```python
from build123d import *

# Parameters (mm, degrees)
SKETCH1_R               = 22
BOSS_EXTRUDE1_DEPTH     = 8.25
SKETCH2_R               = 18
CUT_EXTRUDE1_DEPTH      = 13.5
SKETCH3_R               = 19.5
CUT_EXTRUDE2_DEPTH      = 8
CUT_EXTRUDE3_DEPTH      = 36.217183306
CUT_EXTRUDE3_DEPTH_BACK = 36.217183306
SKETCH4_R               = 10
SKETCH6_W               = 3.4
SKETCH6_H               = 2.2
CUT_EXTRUDE5_DEPTH      = 8
CIRPATTERN1_COUNT       = 4
CUT_EXTRUDE6_START      = -1.5
SKETCH7_R               = 22
CUT_EXTRUDE6_DEPTH      = 1.5
CHAMFER1_SIZE           = 1
BOSS_EXTRUDE2_START     = 5
BOSS_EXTRUDE2_DEPTH     = 5
SKETCH9_W               = 10
SKETCH9_H               = 5
CUT_EXTRUDE7_DEPTH      = 37.986484018
SKETCH10_R              = 1
CUT_EXTRUDE8_DEPTH      = 42.764967377


with BuildPart() as part:
    # Sketch1 → Boss-Extrude1 (new, symmetric)
    with BuildSketch(Plane.XY):
        Circle(SKETCH1_R)
    extrude(amount=BOSS_EXTRUDE1_DEPTH, both=True)

    # Sketch2 → Cut-Extrude1 (cut)
    with BuildSketch(Plane.XY.offset(8.25)):
        Circle(SKETCH2_R)
    extrude(amount=-CUT_EXTRUDE1_DEPTH, mode=Mode.SUBTRACT)

    # Sketch3 → Cut-Extrude2 (cut)
    with BuildSketch(Plane.XY.offset(8.25)):
        Circle(SKETCH3_R)
    extrude(amount=-CUT_EXTRUDE2_DEPTH, mode=Mode.SUBTRACT)

    # Sketch4 → Cut-Extrude3 (cut, two sides: drawn at the far end of the back side and taken through both)
    with BuildSketch(Plane(origin=(0, 0, -8.25), x_dir=(-1, 0, 0), z_dir=(0, 0, -1)).offset(-CUT_EXTRUDE3_DEPTH_BACK)):
        with Locations(Location((0, 0, 0), (0, 0, 180))):
            Circle(SKETCH4_R)
    extrude(amount=CUT_EXTRUDE3_DEPTH + CUT_EXTRUDE3_DEPTH_BACK, mode=Mode.SUBTRACT)

    # Sketch6 → Cut-Extrude5 (cut)
    with BuildSketch(Plane.XY.offset(8.25)):
        with Locations((0, 19.5)):
            Rectangle(SKETCH6_W, SKETCH6_H)
    cut_extrude5 = extrude(amount=-CUT_EXTRUDE5_DEPTH, mode=Mode.SUBTRACT)

    # CirPattern1: Cut-Extrude5 ×4 about axis
    cirpattern1_axis = Axis((0, 0, 0), (0, 0, 1))
    for i in range(1, CIRPATTERN1_COUNT):
        add(cut_extrude5.rotate(cirpattern1_axis, i * 360 / CIRPATTERN1_COUNT), mode=Mode.SUBTRACT)

    # Sketch7 → Cut-Extrude6 (cut)
    with BuildSketch(Plane(origin=(0, 0, -8.25), x_dir=(-1, 0, 0), z_dir=(0, 0, -1)).offset(CUT_EXTRUDE6_START)):
        Circle(SKETCH7_R)
    extrude(amount=CUT_EXTRUDE6_DEPTH, mode=Mode.SUBTRACT)

    # Chamfer1
    chamfer1_edges = [part.edges().sort_by_distance(p)[0] for p in [
        (-22, 0, 8.25),
    ]]
    chamfer(chamfer1_edges, length=CHAMFER1_SIZE)

    # Sketch8 → Boss-Extrude2 (add)
    with BuildSketch(Plane(origin=(0, 0, -6.75), x_dir=(-1, 0, 0), z_dir=(0, 0, -1)).offset(BOSS_EXTRUDE2_START)):
        with BuildLine():
            Line((5, 9), (5, 11.5))
            Line((5, 11.5), (10, 11.5))
            Line((10, 11.5), (10, 15.5))
            Line((10, 15.5), (-10, 15.5))
            Line((-10, 15.5), (-10, 11.5))
            Line((-10, 11.5), (-5, 11.5))
            Line((-5, 11.5), (-5, 9))
            Line((-5, 9), (-4.358898944, 9))
            ThreePointArc((-4.358898944, 9), (0, 10), (4.358898944, 9))
            Line((4.358898944, 9), (5, 9))
        make_face()
    extrude(amount=-BOSS_EXTRUDE2_DEPTH)

    # Sketch9 → Cut-Extrude7 (cut, through all)
    with BuildSketch(Plane(origin=(0, 0, -11.75), x_dir=(-1, 0, 0), z_dir=(0, 0, -1))):
        with Locations((0, 11)):
            Rectangle(SKETCH9_W, SKETCH9_H)
    extrude(amount=-CUT_EXTRUDE7_DEPTH, mode=Mode.SUBTRACT)

    # Sketch10 → Cut-Extrude8 (cut, through all)
    with BuildSketch(Plane.XZ.offset(-11.5)):
        with Locations(Location((-7.5, -9.25, 0), (0, 0, 270))):
            Circle(SKETCH10_R)
        with Locations(Location((7.5, -9.25, 0), (0, 0, 180))):
            Circle(SKETCH10_R)
    extrude(amount=-CUT_EXTRUDE8_DEPTH, mode=Mode.SUBTRACT)


solid = part.part
```
CAD build for the part. Positions are in the model's coordinates, mm. A direction names the side the tool comes from. Round coordinates to 2 decimals unless told otherwise and drop trailing zeros. Loops run counter-clockwise (first coordinate to the right, second up) from the corner with the lowest first, then second, coordinate; pieces in that order, holes last. Notation, with made-up numbers: M 14.25,1 L 32.25,1 A13 cw 32.25,12 Z; hole C -37.75,-26.5 d7. An arc over 180 degrees is marked long. Return JSON: item names as keys, results as strings. Group by question number.
(1) Tool access for faces 4 (the flat face through (-1.7, -20, 4)), 5 (the cylindrical face through (7.63, 13.47, -10.24)), 6 (the flat face through (0, 13.5, -9)): list every direction of +Z, -Z, +X, -X, +Y, -Y with a clear straight run to the whole face (end or side of a thin tool).
(2) Mould opens along X. For faces 1 (the flat face through (-10, 13, -9)), 2 (the flat face through (-5, -9, -6.75)), 3 (the flat face through (-20, -1.7, 4)) say: +X half, -X half, draft (parallel to the pull), parting line (faces both ways), or undercut.
(3) Saw through at B-B, the plane z = 1. List the corners of the cut face in (x, y).
(4) Drop flat-ended pins along their axis: P1, Ø2.5, axis at x = -7.5, z = -9.25, coming from the -Y side; P2, Ø10, axis at y = 7, z = 0.5, coming from the +X side; P3, Ø0.9, axis at x = 20, z = 3.5, coming from the -Y side; P4, Ø18, axis at x = 0, y = 0, coming from the -Z side. Give the stop position or say it passes through.
(5) Saw through at A-A, the plane x = 0. List the corners of the cut face in (y, z).
(6) Wall check: probe 1 along Y at (x, z) = (0, -1.3); probe 2 along Y at (x, z) = (0, -5.8); probe 3 along Z at (x, y) = (7.5, 12.95). Give the ranges that are in metal, low to high. Write a range as [from, to].
(7) Saw through at C-C, the plane x = -7.5. Give the number of separate pieces and of enclosed holes in the cut face, and give its area (3 significant figures).
Answer list:
{
 "1": {"face 4": "+Z", "face 5": "+Y, -Y", "face 6": "+Z, -Z"},
 "2": {"face 1": "-X half", "face 2": "draft", "face 3": "undercut"},
 "3": {"outline": "C 0,0 d44; hole M -20.6,-1.7 L -19.43,-1.7 A19.5 ccw -1.7,-19.43 L -1.7,-20.6 L 1.7,-20.6 L 1.7,-19.43 A19.5 ccw 19.43,-1.7 L 20.6,-1.7 L 20.6,1.7 L 19.43,1.7 A19.5 ccw 1.7,19.43 L 1.7,20.6 L -1.7,20.6 L -1.7,19.43 A19.5 ccw -19.43,1.7 L -20.6,1.7 Z"},
 "4": {"P1": "y = 11.5", "P2": "x = 21.91", "P3": "y = -10.09", "P4": "through"},
 "5": {"outline": "M -22,-6.75 L -10,-6.75 L -10,-5.25 L -18,-5.25 L -18,0.25 L -20.6,0.25 L -20.6,8.25 L -21,8.25 L -22,7.25 Z; M 13.5,-11.75 L 15.5,-11.75 L 15.5,-6.75 L 22,-6.75 L 22,7.25 L 21,8.25 L 20.6,8.25 L 20.6,0.25 L 18,0.25 L 18,-5.25 L 13.5,-5.25 Z"},
 "6": {"probe 1": "[-22, -18], [18, 22]", "probe 2": "[-22, -10], [13.5, 22]", "probe 3": "[-11.75, -10.25], [-8.25, -5.25]"},
 "7": {"separate pieces": "3", "enclosed holes": "0", "area": "144 mm2"}
}
